Here's the drawing with two shaded views (mm, measured from the low corner). I have some questions. Round coordinates to 2 decimals unless told otherwise and drop trailing zeros. Order: outer loops, then holes, each group sorted by start corner. A loop starts at its lowest first (then second) coordinate and runs counter-clockwise, first axis right, second up.
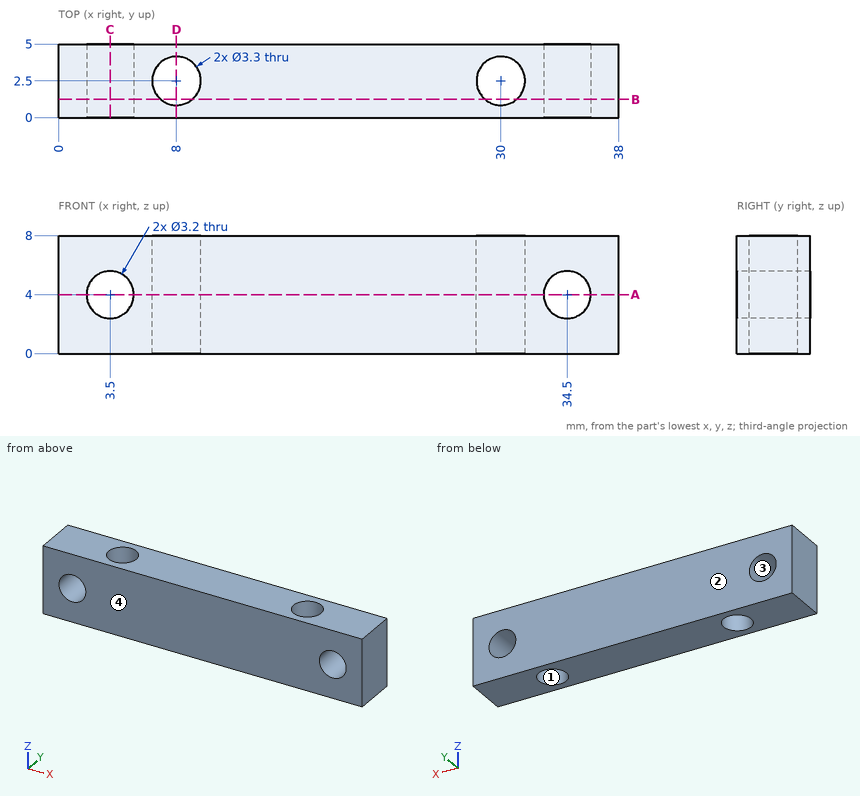
Q1. For P1, Ø3, axis at x = 3.5, z = 4, coming from the +Y side, with a flat end and sliding along its axis, tell me the tip position at first contact or that it passes through.
Q2. Imagine slicing it at A-A, the plane z = 4. Please give me the cut outline in (x, y).
Q3. I need wall thicknesses on L1, parallel to Y at x = 30, z = 3.5; L2, parallel to X at y = 2, z = 5.75; L3, parallel to X at y = 2.7, z = 5.25. Which ranges of each line are inside material? Lowest first, please.
Q4. Imagine slicing it at D-D, the plane x = 8. Please give me the cut outline in (y, z).
Q5. Imagine slicing it at C-C, the plane x = 3.5. Please give me the cut outline in (y, z).
Q6. We'd pull the mould along Y, two halves only. Please class the marked faces 1, 2, 3 and 4: released by +Y, released by -Y, zero draft, split by the parting line, or undercut.
Q7. Imagine slicing it at B-B, the plane y = 1.25. Please give me the cut outline in (x, z), then the cut area to 3 significant figures.
Filled in:
1. P1: passes through
2. outline: (0, 0) - (1.9, 0) - (1.9, 5) - (0, 5) - close; (5.1, 0) - (32.9, 0) - (32.9, 5) - (5.1, 5) - close; (36.1, 0) - (38, 0) - (38, 5) - (36.1, 5) - close; hole circle Ø3.3 at (8, 2.5); hole circle Ø3.3 at (30, 2.5)
3. L1: y = 0 to 0.85, 4.15 to 5
3. L2: x = 0 to 6.43, 9.57 to 28.43, 31.57 to 38
3. L3: x = 0 to 2.5, 4.5 to 6.36, 9.64 to 28.36, 31.64 to 33.5, 35.5 to 38
4. outline: (0, 0) - (0.85, 0) - (0.85, 8) - (0, 8) - close; (4.15, 0) - (5, 0) - (5, 8) - (4.15, 8) - close
5. outline: (0, 0) - (5, 0) - (5, 2.4) - (0, 2.4) - close; (0, 5.6) - (5, 5.6) - (5, 8) - (0, 8) - close
6. face 1: undercut
6. face 2: released by +Y
6. face 3: zero draft
6. face 4: released by -Y
7. outline: (0, 0) - (6.92, 0) - (6.92, 8) - (0, 8) - close; (9.08, 0) - (28.92, 0) - (28.92, 8) - (9.08, 8) - close; (31.08, 0) - (38, 0) - (38, 8) - (31.08, 8) - close; hole circle Ø3.2 at (3.5, 4); hole circle Ø3.2 at (34.5, 4)
7. area: 253 mm2
